The listing builds one solid part. Answer for the finished solid, in the listing's coordinates (mm). Give positions to 0.01 mm unless a question says otherwise; leave off trailing zeros. Order: outer loops, then holes, each group sorted by start corner. A loop starts at its lowest first (then second) coordinate and runs counter-clockwise, first axis right, second up. Notation, with made-up numbers: (56.25, 85.25) - (114.25, 85.25) arc R16 cw to (114.25, 102.25) - close; hole circle Ø1 at (72.25, 4.5). An arc over 180 degrees is marked (long way). Answer in a Markdown table with one row per item.
from build123d import *

# Parameters (mm, degrees)
SKETCH1_W           = 75
SKETCH1_H           = 13
SKETCH1_R           = 2.5
BOSS_EXTRUDE1_DEPTH = 3.175
CUT_EXTRUDE1_DEPTH  = 3.175
FILLET2_R           = 3
FILLET3_R           = 3


with BuildPart() as part:
    # Sketch1 → Boss-Extrude1 (new body)
    with BuildSketch(Plane.XY):
        Rectangle(SKETCH1_W, SKETCH1_H)
        with Locations((33.5, 0)):
            Circle(SKETCH1_R, mode=Mode.SUBTRACT)
        with Locations((9.5, 0)):
            Circle(SKETCH1_R, mode=Mode.SUBTRACT)
    extrude(amount=BOSS_EXTRUDE1_DEPTH)

    # Sketch3 → Cut-Extrude1 (cut)
    with BuildSketch(Plane.XY.offset(3.175)):
        with BuildLine():
            Line((-35.780363842, 6.5), (1.520225121, 6.5))
            add(Edge.make_bspline(
                [(-35.780363842, 6.5), (-18.824487267, -9.098123968), (1.520225121, 6.5)],
                knots=[0, 0, 0, 1, 1, 1], degree=2))
        make_face()
    extrude(amount=-CUT_EXTRUDE1_DEPTH, mode=Mode.SUBTRACT)

    # Fillet2
    fillet2_edges = [part.edges().sort_by_distance(p)[0] for p in [
        (-35.780363842, 6.5, 1.5875),
        (1.520225121, 6.5, 1.5875),
    ]]
    fillet(fillet2_edges, radius=FILLET2_R)

    # Fillet3
    # the kernel refuses this fillet: 3 mm, written as the material it takes off along each edge
    with BuildSketch(Plane(origin=(37.5, -6.5, -7.5), x_dir=(-1, 0, 0), z_dir=(0, 0, 1)), Plane(origin=(-37.5, -6.5, -7.5), x_dir=(0, 1, 0), z_dir=(0, 0, 1)), Plane(origin=(37.5, 6.5, -7.5), x_dir=(0, -1, 0), z_dir=(0, 0, 1))) as fillet3_piece_1:
        with BuildLine():
            CenterArc((FILLET3_R, -FILLET3_R), FILLET3_R, 90, 90)
            Line((0, -FILLET3_R), (-FILLET3_R * 0.02, -FILLET3_R))
            Line((-FILLET3_R * 0.02, -FILLET3_R), (-FILLET3_R * 0.02, FILLET3_R * 0.02))
            Line((-FILLET3_R * 0.02, FILLET3_R * 0.02), (FILLET3_R, FILLET3_R * 0.02))
            Line((FILLET3_R, FILLET3_R * 0.02), (FILLET3_R, 0))
        make_face()
    extrude(amount=18.175, mode=Mode.SUBTRACT)
    with BuildSketch(Plane(origin=(-37.5, 6.5, -4.409176768), x_dir=(1, 0, 0), z_dir=(0, 0, 1))) as fillet3_piece_2:
        with BuildLine():
            CenterArc((3, -1.763670707), FILLET3_R, 143.992564568, 36.007435432)
            Line((0, -1.763670707), (-0.06, -1.763670707))
            Line((-0.06, -1.763670707), (-0.06, 0))
            Line((-0.06, 0), (0, 0.06))
            ThreePointArc((0, 0.06), (0.286588936, 0.06), (0.52464143, 0.035273414))
            Line((0.52464143, 0.035273414), (0.573177873, 0))
        make_face()
    extrude(amount=11.993353536, mode=Mode.SUBTRACT)


solid = part.part
Item 1: This flat-tipped pin is pushed along its axis until it touches: P1, Ø6.5, axis at x = 9.5, y = 0, coming from the -Z side. Where does it stop, or does it pass through?
Answer block:
| item | result |
|---|---|
| P1 | z = 0 |
Item 2: Find section B-B on y = 1. Count the separate pieces of the cut face and the enclosed holes in it, then the cut area to 3 significant figures.
Answer block:
| item | result |
|---|---|
| separate pieces | 4 |
| enclosed holes | 0 |
| area | 145 mm² |
Item 3: Find section A-A on x = 33.5. Write down the section's boundary in (y, z) (3 decimals).
Answer block:
| item | result |
|---|---|
| outline | (-6.5, 0) - (-2.5, 0) - (-2.5, 3.175) - (-6.5, 3.175) - close; (2.5, 0) - (6.5, 0) - (6.5, 3.175) - (2.5, 3.175) - close |
Item 4: Determine the mould class of faces 1 (the face through (36.64, 5.6, 1.57)), 2 (the face through (-1, -1, 0)), 3 (the face through (7, 0, 2)) for opening direction X: pulls with the +X half, pulls with the -X half, needs draft (parallel to the pull), parting line crosses it, or undercut.
Answer block:
| item | result |
|---|---|
| face 1 | pulls with the +X half |
| face 2 | needs draft |
| face 3 | undercut |
Item 5: Consider line 1 (Y direction, x = 33.5, z = 1.3); line 2 (X direction, y = 0.75, z = 2.15); line 3 (Y direction, x = -18, z = 2.4). Determine where each line is inside the solid, lowest interval first.
Answer block:
| item | result |
|---|---|
| line 1 | -6.5 to -2.5, 2.5 to 6.5 |
| line 2 | -37.5 to -27.31, -8.2 to 7.12, 11.88 to 31.12, 35.88 to 37.5 |
| line 3 | -6.5 to -1.3 |
